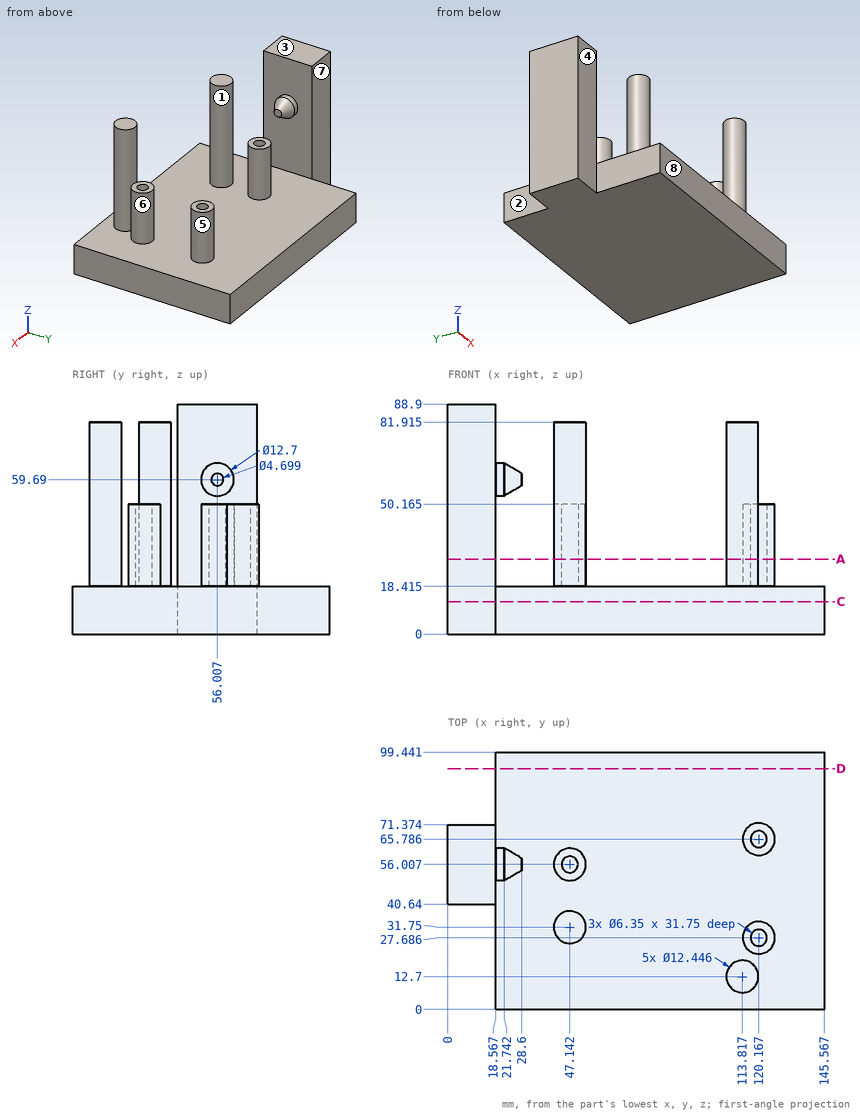
The figure shows three views and two pictorial views of one solid part (mm, origin at its lowest corner). Answer the questions. A direction names the side the tool comes from. Give positions to 0.01 mm unless a question says otherwise; leave off trailing zeros. Loops run counter-clockwise (first coordinate to the right, second up) from the corner with the lowest first, then second, coordinate; pieces in that order, holes last. Notation, with made-up numbers: (8.5, 60.25) -> (33.5, 60.25) arc R10 ccw to (33.5, 72.25) -> close; hole circle Ø1 at (86, 30). An arc over 180 degrees is marked (long way). Use CSV: the item, a comma, the result in double quotes.
1. The part is cut by section A-A (z = 29). State how many separate pieces and enclosed holes the cut face has, then the cut area to 3 significant figures.
Found:
separate pieces,"6"
enclosed holes,"3"
area,"1,080 mm^2"
2. The part is cut by section C-C (z = 12.5). Write down the section's boundary in (x, y), then the cut area to 3 significant figures.
Found:
outline,"(0, 40.64) -> (18.57, 40.64) -> (18.57, 0) -> (145.57, 0) -> (145.57, 99.44) -> (18.57, 99.44) -> (18.57, 71.37) -> (0, 71.37) -> close"
area,"13,200 mm^2"
3. The mould has two halves that part along Y. Classify the marked faces 5, 6, 7 and 8: +Y half, -Y half, draft (parallel to the pull), parting line (faces both ways), or undercut.
Found:
face 5,"undercut"
face 6,"undercut"
face 7,"+Y half"
face 8,"-Y half"
4. Straight lines are drawn through the part: line 1 (X direction, y = 53.5, z = 32) (1 decimal); line 2 (Z direction, x = 86.5, y = 63.5) (1 decimal); line 3 (Y direction, x = 16.5, z = 9.5). For each, find the intervals that lie inside material, in ascending order.
Found:
line 1,"0 to 18.6, 41.4 to 45.2, 49.1 to 52.8"
line 2,"0 to 18.4"
line 3,"40.64 to 71.37"
5. The part is cut by section D-D (y = 93). Write down the section's boundary in (x, z) (1 decimal).
Found:
outline,"(18.6, 0) -> (145.6, 0) -> (145.6, 18.4) -> (18.6, 18.4) -> close"
6. Flat-ended cylindrical pins translate along their axes: pin 1 Ø4 at (x, y) = (100.5, 58) entering from +Z (3 decimals); pin 2 Ø7.5 at (x, y) = (120.17, 65.79) entering from +Z (3 decimals); pin 3 Ø8 at (y, z) = (20.5, 64.5) entering from +X (1 decimal); pin 4 Ø6 at (y, z) = (72, 68) entering from -X. Find the tip coordinate at first contact, or state that the pin passes through.
Found:
pin 1,"z = 18.415"
pin 2,"z = 50.165"
pin 3,"x = 118.7"
pin 4,"x = 0"
7. A tool of negligible diameter and unlimited length cuts with its end or side. For the marked faces 1, 2, 3 and 4, from which of +Z, -Z, +X, -X, +Y, -Y can it reach the whole face along a straight path? Write none if from no direction.
Found:
face 1,"+Z"
face 2,"+Z, -Z, -X, +Y"
face 3,"+Z, +X, -X, +Y, -Y"
face 4,"+Z, -Z, -X, -Y"
